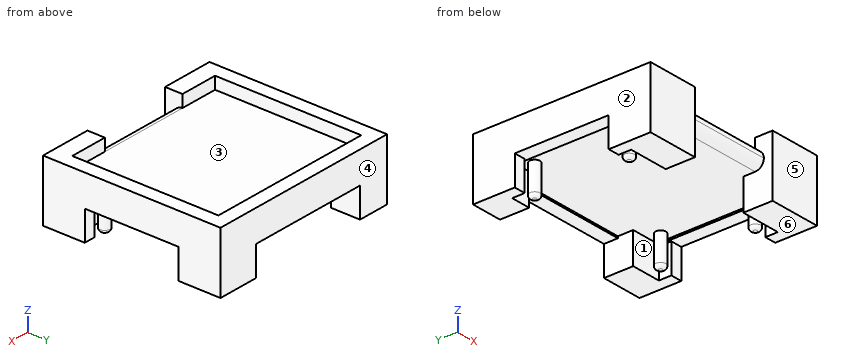
```python
from build123d import *

# Parameters (mm, degrees)
F0_W     = 26.2
F0_H     = 2.5
F1_DEPTH = 5
F2_DEPTH = 8.5
F4_DEPTH = 9
F3_R     = 1.5
F5_DEPTH = 9
F6_R     = 1
F7_R     = 2.49999


# Not quite as in the source:
# - a fillet or chamfer is up to 0.001 mm smaller than in the source, because OpenCascade refuses the exact size


with BuildPart() as f1:
    # F0 (on Top) → F1 (new body)
    with BuildSketch(Plane.XY):
        Polygon((13.1, -20.5), (23.1, -20.5), (24.1, -20.5), (24.1, 21.5), (-24.1, 21.5), (-24.1, -20.5), (-23.1, -20.5), (-13.1, -20.5), align=None)
        with Locations((0, -21.75)):
            Rectangle(F0_W, F0_H)
        Polygon((-13.1, -23), (-13.1, -20.5), (-23.1, -20.5), (-24.1, -20.5), (-28.1, -20.5), (-28.1, -25.5), (-13.1, -25.5), align=None)
    extrude(amount=F1_DEPTH)

    # F0 (on Top) → F2 (join)
    with BuildSketch(Plane.XY):
        Polygon((24.1, -20.5), (23.1, -20.5), (13.1, -20.5), (13.1, -23), (13.1, -25.5), (28.1, -25.5), (28.1, -20.5), align=None)
        Polygon((24.1, 21.5), (24.1, -20.5), (28.1, -20.5), (28.1, 25.5), (-28.1, 25.5), (-28.1, -20.5), (-24.1, -20.5), (-24.1, 21.5), align=None)
        Polygon((-13.1, -23), (-13.1, -20.5), (-23.1, -20.5), (-24.1, -20.5), (-28.1, -20.5), (-28.1, -25.5), (-13.1, -25.5), align=None)
    extrude(amount=F2_DEPTH)

    # F3 (on face) → F4 (join)
    with BuildSketch(Plane(origin=(0, 0, 0), x_dir=(1, 0, 0), z_dir=(0, 0, -1))):
        Polygon((-28.1, 13.5), (-24.75, 13.5), (-24.75, 17.1), (-13.1, 17.1), (-13.1, 23), (-13.1, 25.5), (-28.1, 25.5), align=None)
        Polygon((-19.0010517836, -25.5), (-19.0010517836, -17.1), (-24.75, -17.1), (-24.75, -13.5), (-28.1, -13.5), (-28.1, -25.5), align=None)
        Polygon((24.75, -13.5), (24.75, -17.1), (16.1, -17.1), (16.1, -25.5), (28.1, -25.5), (28.1, -13.5), align=None)
        Polygon((24.75, 17.1), (24.75, 13.5), (28.1, 13.5), (28.1, 25.5), (13.1, 25.5), (13.1, 23), (13.1, 17.1), align=None)
    extrude(amount=F4_DEPTH)

    # F3 (on face) + F2_face1 (on face) → F5 (join)
    with BuildSketch(Plane(origin=(0, 0, 0), x_dir=(1, 0, 0), z_dir=(0, 0, -1))):
        with Locations((-21.25, 13.6)):
            Circle(F3_R)
        with Locations((-21.25, -13.6)):
            Circle(F3_R)
        with Locations((21.25, -13.6)):
            Circle(F3_R)
        with Locations((21.25, 13.6)):
            Circle(F3_R)
    with BuildSketch(Plane(origin=(0, 2.8148564997, 8.5), x_dir=(1, 0, 0), z_dir=(0, 0, 1))):
        Polygon((24.1, -23.3148564997), (13.1, -23.3148564997), (13.1, -28.3148564997), (28.1, -28.3148564997), (28.1, 22.6851435003), (-28.1, 22.6851435003), (-28.1, -28.3148564997), (-13.1, -28.3148564997), (-13.1, -23.3148564997), (-24.1, -23.3148564997), (-24.1, 18.6851435003), (24.1, 18.6851435003), align=None)
    extrude(amount=F5_DEPTH, dir=(0, 0, -1))

    # F6
    f6_edges = [f1.edges().sort_by_distance(p)[0] for p in [
        (-22.75, 13.6, -9),
        (-22.75, -13.6, -9),
        (19.75, -13.6, -9),
        (19.75, 13.6, -9),
    ]]
    fillet(f6_edges, radius=F6_R)

    # F7 (radius 2.5 in the source; OpenCascade refuses exactly that, so slightly less here)
    f7_edges = [f1.edges().sort_by_distance(p)[0] for p in [
        (0, -23, 0),
        (0, -23, 5),
    ]]
    fillet(f7_edges, radius=F7_R)


solid = f1.part
```
Here's how the part is built. I have some questions about the finished solid (model axes, mm). Face numbers are marked on the shaded views. A direction names the side the tool comes from. Coordinates: 2 decimals unless noted, no trailing zeros. Write each loop counter-clockwise with the first axis right and the second up, starting at its lowest first coordinate (ties: lowest second). Pieces come first, ordered by that corner, then holes. Notation, with made-up numbers: (51.25, 86.25) - (107.25, 86.25) arc R24 cw to (107.25, 96.25) - close; hole circle Ø9 at (80, -5.5). An arc over 180 degrees is marked (long way). One line per item, written item: value.
1) I'm going to push flat-ended pins straight in: P1, Ø21, axis at x = 9, y = -2.5, coming from the -Z side; P2, Ø8, axis at x = -5.5, z = -3, coming from the -Y side; P3, Ø1.8, axis at x = -8.5, z = 7.5, coming from the -Y side. Where does each tip first touch, or does it pass through?
Model answer:
P1: stops at z = 0
P2: stops at y = -22.5
P3: stops at y = 21.5
2) On a 3-axis mill with a long thin cutter (end or side, diameter ignored), from which of +Z, -Z, +X, -X, +Y, -Y can I reach the whole of each face in a straight line? I mean the marked faces 1 and 2. Say none if no direction works.
Model answer:
face 1: -Z
face 2: +Z, -Z, -X, +Y, -Y
3) Suppose I cut it at C-C on y = -10. Write out the boundary of the cut face in (x, z).
Model answer:
outline: (-28.1, -0.5) - (-24.1, -0.5) - (-24.1, 0) - (24.1, 0) - (24.1, -0.5) - (28.1, -0.5) - (28.1, 8.5) - (24.1, 8.5) - (24.1, 5) - (-24.1, 5) - (-24.1, 8.5) - (-28.1, 8.5) - close
4) Suppose I cut it at A-A on z = -6.5. Write out the boundary of the cut face in (x, y), and give its area (3 significant figures).
Model answer:
outline: (-28.1, -25.5) - (-13.1, -25.5) - (-13.1, -17.1) - (-24.75, -17.1) - (-24.75, -13.5) - (-28.1, -13.5) - close; (-28.1, 13.5) - (-24.75, 13.5) - (-24.75, 17.1) - (-19, 17.1) - (-19, 25.5) - (-28.1, 25.5) - close; circle Ø3 at (-21.25, -13.6); circle Ø3 at (-21.25, 13.6); (13.1, -25.5) - (28.1, -25.5) - (28.1, -13.5) - (24.75, -13.5) - (24.75, -17.1) - (13.1, -17.1) - close; (16.1, 17.1) - (24.75, 17.1) - (24.75, 13.5) - (28.1, 13.5) - (28.1, 25.5) - (16.1, 25.5) - close; circle Ø3 at (21.25, -13.6); circle Ø3 at (21.25, 13.6)
area: 506 mm²
5) I need wall thicknesses on line 1 along Y through (x, z) = (19.5, -5.5); line 2 along Y through (x, z) = (-14.5, 6); line 3 along Y through (x, z) = (21.5, -5). Which ranges of each line are inside material? Lowest first, please.
Model answer:
line 1: y = -25.5 to -17.1, 17.1 to 25.5
line 2: y = -25.5 to -20.5, 21.5 to 25.5
line 3: y = -25.5 to -17.1, -15.08 to -12.12, 12.12 to 15.08, 17.1 to 25.5
6) We'd pull the mould along Y, two halves only. Please class the marked faces 3, 4, 5 and 6: pulls with the +Y half, pulls with the -Y half, needs draft (parallel to the pull), parting line crosses it, or undercut.
Model answer:
face 3: undercut
face 4: pulls with the +Y half
face 5: pulls with the -Y half
face 6: needs draft
7) Suppose I cut it at D-D on z = 1. Write out the boundary of the cut face in (x, y), and give its area (3 significant figures).
Model answer:
outline: (-28.1, -25.5) - (-13.1, -25.5) - (-13.1, -22.5) - (13.1, -22.5) - (13.1, -25.5) - (28.1, -25.5) - (28.1, 25.5) - (-28.1, 25.5) - close
area: 2,790 mm²
